For this review, take the finished solid that the model builds, in its own axes (mm). A direction names the side the tool comes from. Give positions to 0.01 mm unless a question says otherwise; leave off trailing zeros. Loops run counter-clockwise (first coordinate to the right, second up) from the corner with the lowest first, then second, coordinate; pieces in that order, holes last.
```python
from build123d import *

# Parameters (mm, degrees)
SKETCH1_W             = 50
SKETCH1_H             = 40
BOSS_EXTRUDE1_DEPTH   = 81
SKETCH2_R             = 15
BOSS_EXTRUDE2_DEPTH   = 81
SKETCH3_R             = 2.5
CUT_EXTRUDE1_DEPTH    = 41
M6_TAPPED_HOLE1_D     = 5
M6_TAPPED_HOLE1_DEPTH = 13.497848452
M6_TAPPED_HOLE1_TIP   = 1.502151548
M6_TAPPED_HOLE4_D     = 5
M6_TAPPED_HOLE4_DEPTH = 13.497848452
M6_TAPPED_HOLE4_TIP   = 1.502151548


with BuildPart() as part:
    # Sketch1 → Boss-Extrude1 (new body)
    with BuildSketch(Plane(origin=(0, 0, 0), x_dir=(1, 0, 0), z_dir=(0, 1, 0))):
        with Locations((25, 20)):
            Rectangle(SKETCH1_W, SKETCH1_H)
    extrude(amount=BOSS_EXTRUDE1_DEPTH)

    # Sketch2 → Boss-Extrude2 (add)
    with BuildSketch(Plane.XZ):
        with Locations((25, -20)):
            Circle(SKETCH2_R)
    extrude(amount=BOSS_EXTRUDE2_DEPTH)

    # Sketch3 → Cut-Extrude1 (cut, through all)
    with BuildSketch(Plane.XY):
        with Locations((25, -40.5)):
            Circle(SKETCH3_R)
    extrude(amount=-CUT_EXTRUDE1_DEPTH, mode=Mode.SUBTRACT)

    # M6 Tapped Hole1
    with Locations(Plane.XY):
        with Locations((10, 10), (40, 10), (40, 71), (10, 71)):
            Hole(M6_TAPPED_HOLE1_D / 2, depth=M6_TAPPED_HOLE1_DEPTH)
            with Locations((0, 0, -(M6_TAPPED_HOLE1_DEPTH + M6_TAPPED_HOLE1_TIP / 2))):  # 118° drill point
                Cone(0, M6_TAPPED_HOLE1_D / 2, M6_TAPPED_HOLE1_TIP, mode=Mode.SUBTRACT)

    # M6 Tapped Hole4
    with Locations(Plane(origin=(50.277007324, 10.627759916, -40), x_dir=(-1, 0, 0), z_dir=(0, 0, -1))):
        with Locations((10.277007324, -0.627759916), (40.277007324, -0.627759916), (40.277007324, 60.372240084), (10.277007324, 60.372240084)):
            Hole(M6_TAPPED_HOLE4_D / 2, depth=M6_TAPPED_HOLE4_DEPTH)
            with Locations((0, 0, -(M6_TAPPED_HOLE4_DEPTH + M6_TAPPED_HOLE4_TIP / 2))):  # 118° drill point
                Cone(0, M6_TAPPED_HOLE4_D / 2, M6_TAPPED_HOLE4_TIP, mode=Mode.SUBTRACT)


solid = part.part
```
Item 1: Take a section at B-B on z = -7.5. Give the boundary of the cut face in (x, y).
Answer:
outline: (0, 0) - (16.71, 0) - (16.71, -81) - (33.29, -81) - (33.29, 0) - (50, 0) - (50, 81) - (0, 81) - close; hole circle Ø5 at (10, 10); hole circle Ø5 at (10, 71); hole circle Ø5 at (25, -40.5); hole circle Ø5 at (40, 10); hole circle Ø5 at (40, 71)
Item 2: Take a section at A-A on x = 25. Give the boundary of the cut face in (y, z).
Answer:
outline: (-81, -35) - (-43, -35) - (-43, -5) - (-81, -5) - close; (-38, -35) - (0, -35) - (0, -40) - (81, -40) - (81, 0) - (0, 0) - (0, -5) - (-38, -5) - close
Item 3: Take a section at D-D on y = -34. Give the boundary of the cut face in (x, z), and give its area (3 significant figures).
Answer:
outline: circle Ø30 at (25, -20)
area: 707 mm2
Item 4: The part is to be moulded in two halves that separate along X. For faces 4 (the flat face through (0, 40, -20)), 5 (the flat face through (25, -81, -20)), 6 (the cylindrical face through (10.54, 68.56, -6.84)), say which applies: released by +X, released by -X, zero draft, split by the parting line, or undercut.
Answer:
face 4: released by -X
face 5: zero draft
face 6: undercut
Item 5: Clearance check with flat-ended pins moving along their axes: pin 1 Ø3 at (x, y) = (25, -40.5) entering from -Z; pin 2 Ø10 at (y, z) = (-55, -15.5) entering from +X; pin 3 Ø4 at (x, y) = (40, 71) entering from +Z; pin 4 Ø4.5 at (x, y) = (10, 10) entering from +Z. State where each tip first meets the part, or that it passes through.
Answer:
pin 1: passes through
pin 2: stops at x = 40
pin 3: stops at z = -13.8
pin 4: stops at z = -13.65
Item 6: Tool access review of faces 1 (the cylindrical face through (24.46, -42.94, -19.79)), 2 (the cylindrical face through (42.31, 70.04, -33.16)), 3 (the cylindrical face through (10.54, 7.56, -6.84)): name each direction out of +Z, -Z, +X, -X, +Y, -Y from which nothing blocks a thin tool from reaching the whole face with its end or side.
Answer:
face 1: +Z, -Z
face 2: -Z
face 3: +Z
Item 7: For L1, parallel to X at y = 10, z = -5; L2, parallel to Y at x = 10, z = -5; L3, parallel to X at y = -10, z = -19, list the stretches that pass through material, from the lowest coordinate up.
Answer:
L1: x = 0 to 7.5, 12.5 to 37.5, 42.5 to 50
L2: y = 0 to 7.5, 12.5 to 68.5, 73.5 to 81
L3: x = 10.03 to 39.97
Item 8: Take a section at C-C on x = 17. Give the boundary of the cut face in (y, z).
Answer:
outline: (-81, -32.69) - (0, -32.69) - (0, -40) - (81, -40) - (81, 0) - (0, 0) - (0, -7.31) - (-81, -7.31) - close
